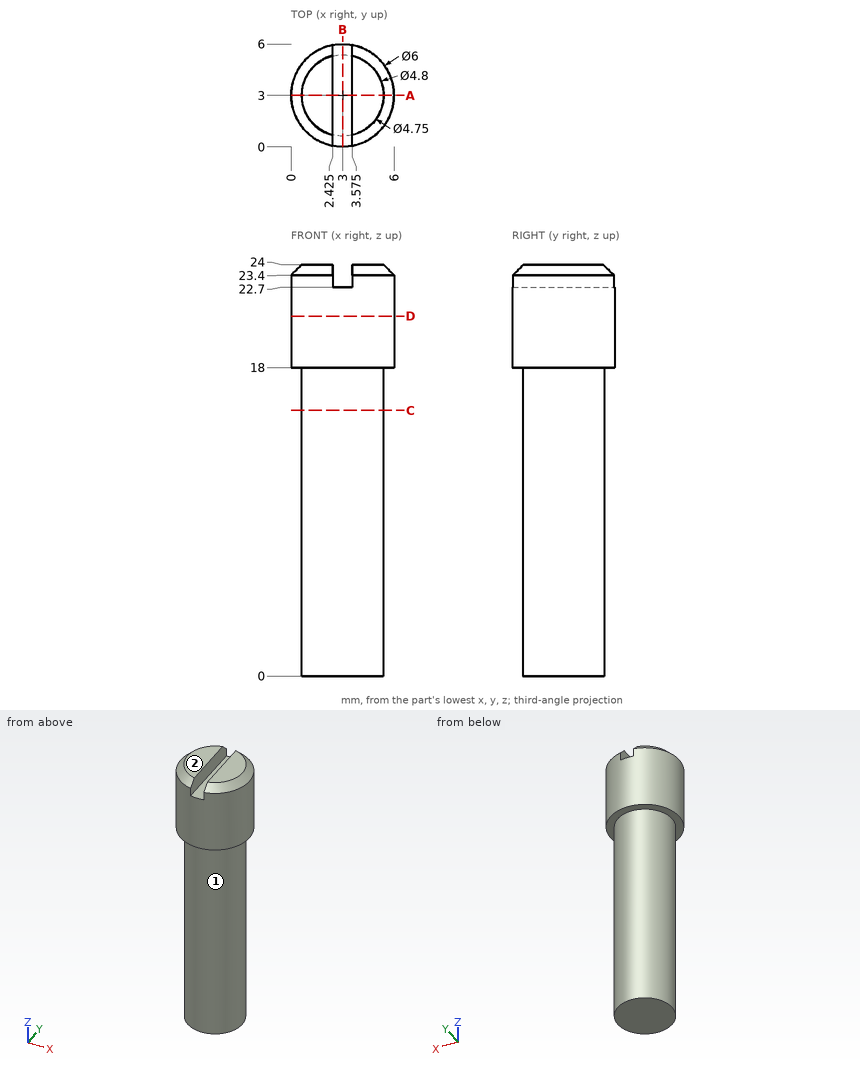
For this review, use the dimensioned drawing (mm, ordinates from the lowest corner) and the shaded views. A direction names the side the tool comes from. Coordinates: 2 decimals unless noted, no trailing zeros. Loops run counter-clockwise (first coordinate to the right, second up) from the corner with the lowest first, then second, coordinate; pieces in that order, holes last. Notation, with made-up numbers: (23.25, -1.5) -> (28.25, -1.5) arc R9 ccw to (28.25, 15.5) -> close; hole circle Ø2 at (69, 7). An arc over 180 degrees is marked (long way). Return JSON: item names as keys, results as strings. Group by question number.
(1) To check wall thickness, follow L1, parallel to Z at x = 3.1, y = 2.4; L2, parallel to Y at x = 2.85, z = 7.75; L3, parallel to Z at x = 5, y = 1.65. State the ranges of each line that lie inside material, in increasing order.
(2) Consider section D-D, the plane z = 21. Give the boundary of the cut face in (x, y), plus the area to 3 significant figures.
(3) Consider section B-B, the plane x = 3. Give the boundary of the cut face in (y, z) (3 decimals).
(4) Tool access review of the marked faces 1 and 2: name each direction out of +Z, -Z, +X, -X, +Y, -Y from which nothing blocks a thin tool from reaching the whole face with its end or side.
(5) For pin 1 Ø3 at (x, z) = (2.5, 5.5) entering from -Y (3 decimals); pin 2 Ø1 at (y, z) = (4.5, 5.5) entering from -X; pin 3 Ø1 at (y, z) = (2, 23.5) entering from +X, all flat-tipped, find the tip position at first contact; note any pin that passes through.
(6) Consider section C-C, the plane z = 15.5. Give the boundary of the cut face in (x, y) (3 decimals), plus the area to 3 significant figures.
(7) Consider section A-A, the plane y = 3. Give the boundary of the cut face in (x, z) (3 decimals).
Results below:
{
 "1": {"L1": "z = 0 to 22.7", "L2": "y = 0.63 to 5.37", "L3": "z = 18 to 23.99"},
 "2": {"outline": "circle Ø6 at (3, 3)", "area": "28.3 mm2"},
 "3": {"outline": "(0, 18) -> (0.625, 18) -> (0.625, 0) -> (5.375, 0) -> (5.375, 18) -> (6, 18) -> (6, 22.7) -> (0, 22.7) -> close"},
 "4": {"face 1": "-Z", "face 2": "+Z, +X, -X, +Y, -Y"},
 "5": {"pin 1": "stops at y = 0.625", "pin 2": "stops at x = 0.85", "pin 3": "stops at x = 5.96"},
 "6": {"outline": "circle Ø4.75 at (3, 3)", "area": "17.7 mm2"},
 "7": {"outline": "(0, 18) -> (0.625, 18) -> (0.625, 0) -> (5.375, 0) -> (5.375, 18) -> (6, 18) -> (6, 23.4) -> (5.4, 24) -> (3.575, 24) -> (3.575, 22.7) -> (2.425, 22.7) -> (2.425, 24) -> (0.6, 24) -> (0, 23.4) -> close"}
}
